Autodesk Inventor part; units mm, degrees
ref_plane "YZ Plane" through (0, 0, 0) normal (1, 0, 0) x (0, 1, 0)
ref_plane "XZ Plane" through (0, 0, 0) normal (0, 1, 0) x (-1, 0, 0)
ref_plane "XY Plane" through (0, 0, 0) normal (0, 0, 1) x (1, 0, 0)
sketch "Sketch1" plane through (0, 0, 0) normal (0, 0, 1) x (1, 0, 0)
  arc A0 (26.2029, 65.6915) -> (-2.973, 3.4018) centre (110.991, -12) ccw
  line L0 (26.991, 71.9374) -> (26.991, 67.7183)
  arc A1 (26.2029, 65.6915) -> (26.991, 67.7183) centre (23.991, 67.7183) ccw
  arc A2 (29.116, 73.9335) -> (26.991, 71.9374) centre (28.991, 71.9374) ccw
  arc A3 (58.0589, 53.8125) -> (29.116, 73.9335) centre (26.991, 40) ccw
  arc A4 (56.2314, 51) -> (58.0589, 53.8125) centre (56.2314, 53) ccw
  line L1 (53.8596, 51) -> (56.2314, 51)
  arc A5 (53.8596, 51) -> (45.0701, 45.7692) centre (53.8596, 41) ccw
  arc A6 (45.0701, 45.7692) -> (36.2936, 3.2692) centre (110.991, 10) ccw
  arc A7 (33.3057, 0) -> (36.2936, 3.2692) centre (33.3057, 3) ccw
  line L2 (0, 0) -> (33.3057, 0)
  arc A8 (-2.973, 3.4018) -> (0, 0) centre (0, 3) ccw
extrude "Extrusion1" add sketch "Sketch1" along normal blind 6
fillet "Fillet1" radius 2 12 edges at (57.9084, 51.9103, 0) (46.3986, 67.9167, 0) (27.6217, 73.3952, 0) (26.991, 69.8278, 0) (26.787, 66.631, 0) (6.8488, 36.7791, 0) (-2.2589, 1.0258, 0) (16.6529, 0, 0) (35.5202, 0.9761, 0) (37.5408, 25.1679, 0) (48.7455, 49.5934, 0) (55.0455, 51, 0)
sketch "Sketch2" plane through (0, 0, 6) normal (0, 0, 1) x (1, 0, 0)
  circle A0 centre (16.991, 15) radius 5
  circle A1 centre (26.991, 40) radius 5
  circle A2 centre (16.991, 15) radius 2.1
  circle A3 centre (26.991, 40) radius 2.1
  point P0 (0, 0)
extrude "Extrusion2" add sketch "Sketch2" along normal blind 6
chamfer "Chamfer1" distance 1 angle 45 2 edges at (21.991, 40, 12) (11.991, 15, 12)
chamfer "Chamfer2" distance 2 angle 45 1 edges at (24.891, 40, 6)
chamfer "Chamfer3" distance 2 angle 45 1 edges at (14.891, 15, 6)
properties part number "Rukohvat_Levi_2"
For this review, take the finished solid that the model builds, in its own axes (mm). A direction names the side the tool comes from. Give positions to 0.01 mm unless a question says otherwise; leave off trailing zeros. Answer as a JSON object with one key per item and string values. Group by question number.
Item 1: Machinability: for faces 1 (the cylindrical face through (21.996, 39.78, 8.465)), 2 (the cylindrical face through (55.06, 51.57, 0.6)), 3 (the flat face through (55, 51, 4)), which of the approach directions +Z, -Z, +X, -X, +Y, -Y give a long, thin tool a straight path to every point of the face, cutting with its end or side? Answer none if there is none.
Item 2: Wall thickness on line 1 along Z through (x, y) = (25, 60); line 2 along X through (y, z) = (41.5, 11); line 3 along Y through (x, z) = (15.5, 5.25): over which ranges is each line inside the solid? List them lowest first.
Item 3: Clearance check with flat-ended pins moving along their axes: pin 1 Ø6 at (x, y) = (38, 14.5) entering from +Z; pin 2 Ø4 at (x, y) = (16.991, 15) entering from +Z; pin 3 Ø3 at (y, z) = (14.5, 7) entering from +X; pin 4 Ø4 at (y, z) = (23, 9.5) entering from +X. State where each tip first meets the part, or that it passes through.
Item 4: Draft analysis for pull direction Y (two halves, no side actions). For faces 4 (the cylindrical face through (37.48, 24.87, 3.97)), 5 (the flat face through (20, 37, 6)), 6 (the flat face through (16, 0, 4)), state which applies: pulls with the +Y half, pulls with the -Y half, needs draft (parallel to the pull), parting line crosses it, or undercut.
Reported:
{
 "1": {"face 1": "+Z", "face 2": "-Z, +X, -Y", "face 3": "+Z, -Z, +X, -Y"},
 "2": {"line 1": "0 to 6", "line 2": "22.22 to 25.52, 28.46 to 31.76", "line 3": "0 to 52.08"},
 "3": {"pin 1": "z = 6", "pin 2": "z = 7.9", "pin 3": "x = 36.2", "pin 4": "through"},
 "4": {"face 4": "undercut", "face 5": "needs draft", "face 6": "pulls with the -Y half"}
}
